Read the model definition and answer for the solid it produces. Units are mm, in the model's axes. Face numbers are marked on the shaded views. A direction names the side the tool comes from. Give positions to 0.01 mm unless a question says otherwise; leave off trailing zeros. Order: outer loops, then holes, each group sorted by start corner. A loop starts at its lowest first (then second) coordinate and runs counter-clockwise, first axis right, second up.
Item 1: A cutting plane is placed at A-A (z = 0). Write down the section's boundary in (x, y), plus the area to 3 significant figures.
Item 2: Which of the six approach directions +Z, -Z, +X, -X, +Y, -Y give full straight-line access (tool end or side, diameter ignored) to the marked faces 1, 2 and 3?
Item 3: Given pin 1 Ø4 at (x, z) = (38.5, 16.5) entering from +Y; pin 2 Ø12 at (x, y) = (72.5, -8.5) entering from +Z; pin 3 Ø10 at (x, z) = (121, -14.5) entering from -Y, each flat-ended and moving along its own axis, determine where each tip first touches the part or whether it passes through.
Item 4: Find the intervals of material crossed by line 1 along Z through (x, y) = (145.5, -1); line 2 along X through (y, z) = (-7.5, 43); line 3 along X through (y, z) = (28, -20.5), in increasing order.
Item 5: A cutting plane is placed at C-C (x = 72.5). Write down the section's boundary in (y, z), plus the area to 3 significant figures.
Item 6: A cutting plane is placed at D-D (x = 147). Write down the section's boundary in (y, z), plus the area to 3 significant figures.
Autodesk Inventor part; units mm, degrees
ref_plane "YZ Plane" through (0, 0, 0) normal (1, 0, 0) x (0, 1, 0)
ref_plane "XZ Plane" through (0, 0, 0) normal (0, 1, 0) x (-1, 0, 0)
ref_plane "XY Plane" through (0, 0, 0) normal (0, 0, 1) x (1, 0, 0)
sketch "Skizze1" plane through (0, 0, 0) normal (0, 0, 1) x (1, 0, 0)
  line L0 (0, 0) -> (184, 0)
  line L1 (0, 0) -> (0, 28)
  line L2 (0, 28) -> (84, 28)
  line L3 (84, 28) -> (84, 47)
  line L4 (84, 47) -> (124, 47)
  line L5 (124, 47) -> (124, 35)
  line L6 (124, 35) -> (154, 35)
  line L7 (154, 35) -> (154, 20)
  line L8 (154, 20) -> (174, 20)
  line L9 (174, 20) -> (174, 15)
  line L10 (174, 15) -> (180, 15)
  line L11 (180, 15) -> (180, 20)
  line L12 (180, 20) -> (184, 20)
  line L13 (184, 20) -> (184, 0)
  dimension "d0" = 184
  dimension "d1" = 4
  dimension "d2" = 20
  dimension "d3" = 30
  dimension "d4" = 40
  dimension "d5" = 40
  dimension "d6" = 30
  dimension "d7" = 84
  dimension "d8" = 56
  dimension "d9" = 94
  dimension "d10" = 70
revolve "Umdrehung1" add sketch "Skizze1" angle 360 about axis through (0, 0, 0) along (1, 0, 0)
chamfer "Fasen1" distance 4 angle 10 1 edges at (0, -28, 0) measured on face at (0, 6.9861, 6.1891)
chamfer "Fasen2" distance 3 angle 45 1 edges at (84, -47, 0)
properties part number "Welle" material "Stahl, galvanisiert"
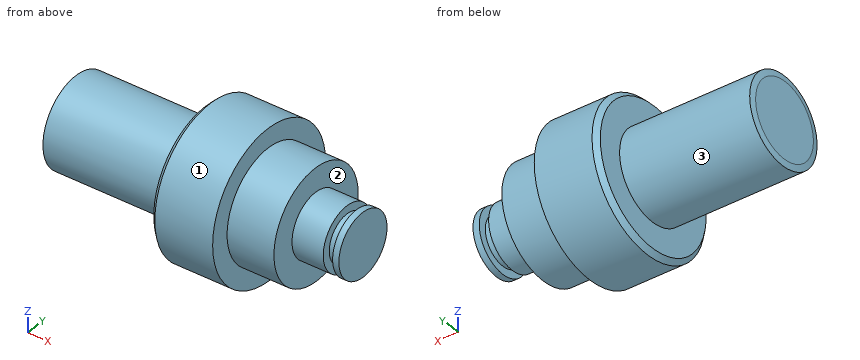
Response values:
1. outline: (0, -24) - (0.71, -28) - (84, -28) - (84, -44) - (87, -47) - (124, -47) - (124, -35) - (154, -35) - (154, -20) - (174, -20) - (174, -15) - (180, -15) - (180, -20) - (184, -20) - (184, 20) - (180, 20) - (180, 15) - (174, 15) - (174, 20) - (154, 20) - (154, 35) - (124, 35) - (124, 47) - (87, 47) - (84, 44) - (84, 28) - (0.71, 28) - (0, 24) - close
1. area: 11,700 mm2
2. face 1: +X, -X
2. face 2: +X
2. face 3: -X
3. pin 1: stops at y = 23.95
3. pin 2: stops at z = 27.89
3. pin 3: stops at y = -46.03
4. line 1: z = -34.99 to 34.99
4. line 2: x = 84 to 124
4. line 3: x = 84 to 154
5. outline: circle Ø56 at (0, 0)
5. area: 2,460 mm2
6. outline: circle Ø70 at (0, 0)
6. area: 3,850 mm2
